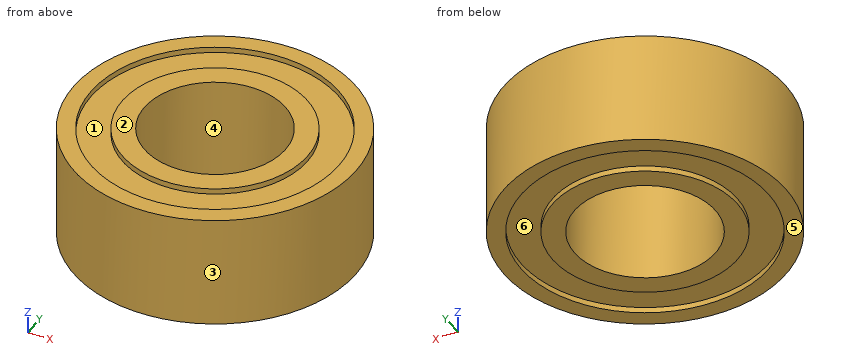
from build123d import *

# Parameters (mm, degrees)
SKETCH1_R           = 5
SKETCH1_R_2         = 2.5
BOSS_EXTRUDE1_DEPTH = 2
SKETCH2_R           = 4.39
SKETCH2_R_2         = 3.28
CUT_EXTRUDE1_DEPTH  = 0.2


with BuildPart() as part:
    # Sketch1 → Boss-Extrude1 (new body, symmetric)
    with BuildSketch(Plane.XY):
        Circle(SKETCH1_R)
        Circle(SKETCH1_R_2, mode=Mode.SUBTRACT)
    extrude(amount=BOSS_EXTRUDE1_DEPTH, both=True)

    # Sketch2 → Cut-Extrude1 (cut)
    with BuildSketch(Plane.XY.offset(2)):
        Circle(SKETCH2_R)
        Circle(SKETCH2_R_2, mode=Mode.SUBTRACT)
    cut_extrude1 = extrude(amount=-CUT_EXTRUDE1_DEPTH, mode=Mode.SUBTRACT)

    # Mirror1: Cut-Extrude1 across plane
    add(cut_extrude1.mirror(Plane.XY), mode=Mode.SUBTRACT)


solid = part.part
Read the model definition and answer for the solid it produces. Units are mm, in the model's axes. Face numbers are marked on the shaded views. A direction names the side the tool comes from. Round coordinates to 2 decimals unless told otherwise and drop trailing zeros. Loops run counter-clockwise (first coordinate to the right, second up) from the corner with the lowest first, then second, coordinate; pieces in that order, holes last.
Q1. Each of these flat-tipped pins is pushed along its axis until it touches: pin 1 (6 mm diameter, centred on x = 0, y = 0, fed in from -Z); pin 2 (2 mm diameter, centred on y = -4, z = 1, fed in from +X); pin 3 (2 mm diameter, centred on x = -2.5, z = -1, fed in from +Y). Where does it stop, or does it pass through?
Q2. Which of the six approach directions +Z, -Z, +X, -X, +Y, -Y give full straight-line access (tool end or side, diameter ignored) to the marked faces 5 and 6?
Q3. Consider probe 1 along Y at (x, z) = (0, -1.9); probe 2 along Y at (x, z) = (0, 0.8); probe 3 along Z at (x, y) = (3, -2.25). Determine where each line is inside the solid, lowest interval first.
Q4. Section A-A on y = 0 is taken. Write down the section's boundary in (x, z).
Q5. Section C-C on z = -1.5 is taken. Write down the section's boundary in (x, y), and give its area (3 significant figures).
Q6. Determine the mould class of the marked faces 1, 2, 3 and 4 for opening direction X: released by +X, released by -X, zero draft, split by the parting line, or undercut.
Output:
1. pin 1: stops at z = -2
1. pin 2: stops at x = 4
1. pin 3: stops at y = 4.77
2. face 5: -Z, +X, -X, +Y, -Y
2. face 6: -Z
3. probe 1: y = -5 to -4.39, -3.28 to -2.5, 2.5 to 3.28, 4.39 to 5
3. probe 2: y = -5 to -2.5, 2.5 to 5
3. probe 3: z = -1.8 to 1.8
4. outline: (-5, -2) - (-4.39, -2) - (-4.39, -1.8) - (-3.28, -1.8) - (-3.28, -2) - (-2.5, -2) - (-2.5, 2) - (-3.28, 2) - (-3.28, 1.8) - (-4.39, 1.8) - (-4.39, 2) - (-5, 2) - close; (2.5, -2) - (3.28, -2) - (3.28, -1.8) - (4.39, -1.8) - (4.39, -2) - (5, -2) - (5, 2) - (4.39, 2) - (4.39, 1.8) - (3.28, 1.8) - (3.28, 2) - (2.5, 2) - close
5. outline: circle Ø10 at (0, 0); hole circle Ø5 at (0, 0)
5. area: 58.9 mm2
6. face 1: undercut
6. face 2: zero draft
6. face 3: split by the parting line
6. face 4: undercut
